Here's how the part is built. I have some questions about the finished solid (model axes, mm). Face numbers are marked on the shaded views. A direction names the side the tool comes from. Coordinates: 2 decimals unless noted, no trailing zeros. Loops run counter-clockwise (first coordinate to the right, second up) from the corner with the lowest first, then second, coordinate; pieces in that order, holes last. Notation, with made-up numbers: (55, 71.5) -> (90, 71.5) arc R31 cw to (90, 104.5) -> close; hole circle Ø9 at (64.5, 5). An arc over 180 degrees is marked (long way). Answer as a JSON object with one key per item and string values. Group by question number.
Q1. I want a section at D-D on x = 17.5. Write out the boundary of the cut face in (y, z).
Q2. Thinking about a two-plate mould opening in Z: for the marked faces 4, 5 and 6, which applies, released by +Z, released by -Z, zero draft, split by the parting line, or undercut?
Q3. I want a section at A-A on z = -5.25. Write out the boundary of the cut face in (x, y), then the cut area to 3 significant figures.
Q4. I need wall thicknesses on line 1 (Z direction, x = 10, y = 2.7); line 2 (Z direction, x = 10, y = 1.7); line 3 (X direction, y = 1.9, z = -5.25). Which ranges of each line are inside material? Lowest first, please.
Q5. On a 3-axis mill with a long thin cutter (end or side, diameter ignored), from which of +Z, -Z, +X, -X, +Y, -Y can I reach the whole of each face in a straight line? I mean the marked faces 1, 2 and 3. Say none if no direction works.
Q6. I want a section at C-C on y = 3.5. Write out the boundary of the cut face in (x, z).
Q7. I want a section at B-B on x = 10. Write out the boundary of the cut face in (y, z).
Q8. I'm going to push flat-ended pins straight in: pin 1 (6 mm diameter, centred on y = 3.5, z = -2.5, fed in from -X); pin 2 (5 mm diameter, centred on x = 10, z = -5.25, fed in from -Y); pin 3 (5 mm diameter, centred on x = 16, z = 27, fed in from -Y); pin 4 (3 mm diameter, centred on x = 11, z = -4, fed in from +Y). Where does each tip first touch, or does it pass through?
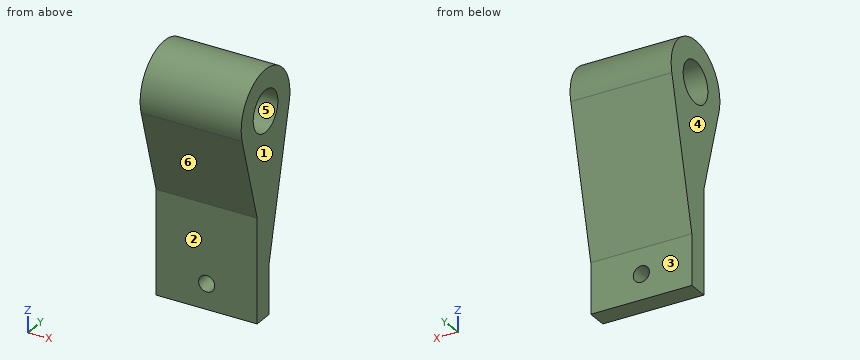
```python
from build123d import *

# Parameters (mm, degrees)
SKETCH1_R           = 4.1
BOSS_EXTRUDE1_DEPTH = 20
SKETCH2_R           = 1.6
CUT_EXTRUDE1_DEPTH  = 10.320966192


with BuildPart() as part:
    # Sketch1 → Boss-Extrude1 (new body)
    with BuildSketch(Plane(origin=(0, 0, 0), x_dir=(0, 0, -1), z_dir=(1, 0, 0))):
        with BuildLine():
            Line((-10.25, 0), (10.25, 0))
            Line((10.25, 0), (10.25, 4))
            Line((10.25, 4), (0.25, 4))
            Line((0.25, 4), (-27.869263808, 10.660915614))
            ThreePointArc((-27.869263808, 10.660915614), (-37.833813874, 2.577122842), (-27.47875844, -5))
            Line((-27.47875844, -5), (-10.25, 0))
        make_face()
        with Locations((-29.736330811, 2.779033808)):
            Circle(SKETCH1_R, mode=Mode.SUBTRACT)
    extrude(amount=BOSS_EXTRUDE1_DEPTH)

    # Sketch2 → Cut-Extrude1 (cut, through all)
    with BuildSketch(Plane(origin=(0, 4, 0), x_dir=(1, 0, 0), z_dir=(0, 1, 0))):
        with Locations((10, 5.25)):
            Circle(SKETCH2_R)
    extrude(amount=-CUT_EXTRUDE1_DEPTH, mode=Mode.SUBTRACT)


solid = part.part
```
Result set:
{
 "1": {"outline": "(-5, 27.48) -> (0, 10.25) -> (0, -10.25) -> (4, -10.25) -> (4, -0.25) -> (10.66, 27.87) arc R8.1 ccw (long way) to start; hole circle Ø8.2 at (2.78, 29.74)"},
 "2": {"face 4": "zero draft", "face 5": "undercut", "face 6": "released by -Z"},
 "3": {"outline": "(0, 0) -> (8.4, 0) -> (8.4, 4) -> (0, 4) -> close; (11.6, 0) -> (20, 0) -> (20, 4) -> (11.6, 4) -> close", "area": "67.2 mm²"},
 "4": {"line 1": "z = -10.25 to -6.85, -3.65 to 25.64, 33.84 to 37.84", "line 2": "z = -10.25 to -6.85, -3.65 to 25.78, 33.69 to 37.76", "line 3": "x = 0 to 8.4, 11.6 to 20"},
 "5": {"face 1": "+Z, -Z, +X, +Y, -Y", "face 2": "-Z, +X, -X, -Y", "face 3": "-Z, +X, -X, +Y"},
 "6": {"outline": "(0, -10.25) -> (20, -10.25) -> (20, 25.7) -> (0, 25.7) -> close; (0, 33.77) -> (20, 33.77) -> (20, 37.8) -> (0, 37.8) -> close; hole circle Ø3.2 at (10, -5.25)"},
 "7": {"outline": "(-5, 27.48) -> (0, 10.25) -> (0, -3.65) -> (4, -3.65) -> (4, -0.25) -> (10.66, 27.87) arc R8.1 ccw (long way) to start; (0, -10.25) -> (4, -10.25) -> (4, -6.85) -> (0, -6.85) -> close; hole circle Ø8.2 at (2.78, 29.74)"},
 "8": {"pin 1": "stops at x = 0", "pin 2": "stops at y = 0", "pin 3": "stops at y = -5.32", "pin 4": "stops at y = 4"}
}
